Read the model definition and answer for the solid it produces. Units are mm, in the model's axes. A direction names the side the tool comes from. Round coordinates to 2 decimals unless told otherwise and drop trailing zeros. Order: outer loops, then holes, each group sorted by start corner. A loop starts at its lowest first (then second) coordinate and runs counter-clockwise, first axis right, second up. Notation, with made-up numbers: M -18.75,-8.75 L 1.25,-8.75 A22 cw 1.25,20.25 Z; hole C 60.5,35 d8. An arc over 180 degrees is marked long. Answer as CSV lines item,"result".
```python
from build123d import *

# Parameters (mm, degrees)
SKETCH_2_R      = 1.1
SKETCH_2_R_2    = 1.6
EXTRUDE_1_DEPTH = 3
FILLET_1_R      = 1


with BuildPart() as part:
    # 草图2 → 凸台-拉伸1 (new body)
    with BuildSketch(Plane.XY):
        Polygon((28, 18.5), (28, 13.5), (-7, 13.5), (-7, -13.5), (28, -13.5), (28, -18.5), (-28, -18.5), (-28, 18.5), align=None)
        with Locations((25, 15.5)):
            Circle(SKETCH_2_R, mode=Mode.SUBTRACT)
        with Locations(Location((25, -15.5, 0), (0, 0, 180))):
            Circle(SKETCH_2_R, mode=Mode.SUBTRACT)
        with Locations((-25, 15.5)):
            Circle(SKETCH_2_R_2, mode=Mode.SUBTRACT)
        with Locations((-15, 15.5)):
            Circle(SKETCH_2_R_2, mode=Mode.SUBTRACT)
        with Locations(Location((-15, -15.5, 0), (0, 0, 180))):
            Circle(SKETCH_2_R_2, mode=Mode.SUBTRACT)
        with Locations(Location((-25, -15.5, 0), (0, 0, 180))):
            Circle(SKETCH_2_R_2, mode=Mode.SUBTRACT)
    extrude(amount=EXTRUDE_1_DEPTH)

    # 圆角1
    fillet_1_edges = [part.edges().sort_by_distance(p)[0] for p in [
        (28, 18.5, 1.5),
        (28, -18.5, 1.5),
        (-28, -18.5, 1.5),
        (-28, 18.5, 1.5),
    ]]
    fillet(fillet_1_edges, radius=FILLET_1_R)


solid = part.part
```
Item 1: Determine the mould class of faces 3 (the face through (0, 18.5, 1)), 4 (the face through (-16.18, 16.58, 1.48)), 5 (the face through (-7, 0, 1)) for opening direction X: +X half, -X half, draft (parallel to the pull), parting line (faces both ways), or undercut.
Ans:
face 3,"draft"
face 4,"undercut"
face 5,"+X half"
Item 2: A tool of negligible diameter and unlimited length cuts with its end or side. For faces 1 (the face through (-26.18, 16.58, 1.48)), 2 (the face through (11, 13.5, 1)), from which of +Z, -Z, +X, -X, +Y, -Y can it reach the whole face along a straight path? Write none if from no direction.
Ans:
face 1,"+Z, -Z"
face 2,"+Z, -Z, +X"
Item 3: Find the intervals of material crossed by probe 1 along X at (y, z) = (-15.5, 2.25); probe 2 along Y at (x, z) = (-15, 0.9); probe 3 along Y at (x, z) = (25, 0.95), in increasing order. Write a range as [from, to].
Ans:
probe 1,"[-28, -26.6], [-23.4, -16.6], [-13.4, 23.9], [26.1, 28]"
probe 2,"[-18.5, -17.1], [-13.9, 13.9], [17.1, 18.5]"
probe 3,"[-18.5, -16.6], [-14.4, -13.5], [13.5, 14.4], [16.6, 18.5]"
Item 4: A cutting plane is placed at B-B, the plane y = 15.5. Determine the outline of the cut face in (x, z).
Ans:
outline,"M -28,0 L -26.6,0 L -26.6,3 L -28,3 Z; M -23.4,0 L -16.6,0 L -16.6,3 L -23.4,3 Z; M -13.4,0 L 23.9,0 L 23.9,3 L -13.4,3 Z; M 26.1,0 L 28,0 L 28,3 L 26.1,3 Z"
Item 5: A cutting plane is placed at A-A, the plane x = 25. Determine the outline of the cut face in (y, z).
Ans:
outline,"M -18.5,0 L -16.6,0 L -16.6,3 L -18.5,3 Z; M -14.4,0 L -13.5,0 L -13.5,3 L -14.4,3 Z; M 13.5,0 L 14.4,0 L 14.4,3 L 13.5,3 Z; M 16.6,0 L 18.5,0 L 18.5,3 L 16.6,3 Z"
Item 6: A cutting plane is placed at C-C, the plane x = -2.5. Determine the outline of the cut face in (y, z), and give its area (3 significant figures).
Ans:
outline,"M -18.5,0 L -13.5,0 L -13.5,3 L -18.5,3 Z; M 13.5,0 L 18.5,0 L 18.5,3 L 13.5,3 Z"
area,"30.0 mm2"
Item 7: A cutting plane is placed at D-D, the plane z = 2.15. Determine the outline of the cut face in (x, y).
Ans:
outline,"M -28,-17.5 A1 ccw -27,-18.5 L 27,-18.5 A1 ccw 28,-17.5 L 28,-13.5 L -7,-13.5 L -7,13.5 L 28,13.5 L 28,17.5 A1 ccw 27,18.5 L -27,18.5 A1 ccw -28,17.5 Z; hole C -25,-15.5 d3.2; hole C -25,15.5 d3.2; hole C -15,-15.5 d3.2; hole C -15,15.5 d3.2; hole C 25,-15.5 d2.2; hole C 25,15.5 d2.2"
